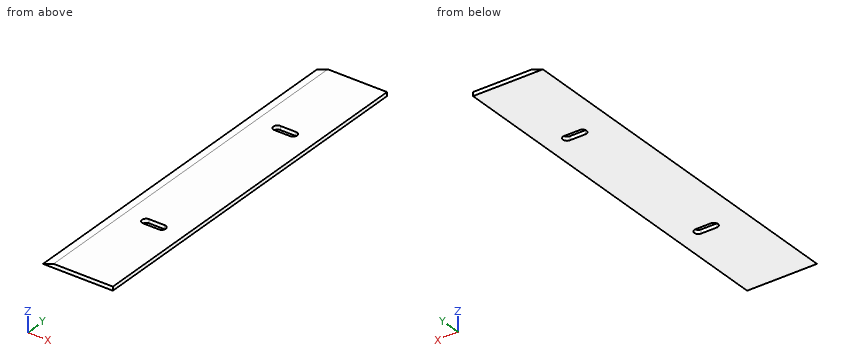
```python
from build123d import *

# Parameters (mm, degrees)
SKETCH_1_W          = 18
SKETCH_1_H          = 96
EXTRUDE_1_DEPTH     = 1
CUT_EXTRUDE_1_DEPTH = 117.756631965


with BuildPart() as part:
    # Эскиз1 → Бобышка-Вытянуть1 (new body)
    with BuildSketch(Plane.XY):
        with Locations((-57.446302439, 0)):
            Rectangle(SKETCH_1_W, SKETCH_1_H)
        with BuildLine():
            Line((-54.254431019, 21.962877229), (-58.271972276, 21.962877229))
            ThreePointArc((-58.271972276, 21.962877229), (-59.309095047, 23), (-58.271972276, 24.037122771))
            Line((-58.271972276, 24.037122771), (-54.254431019, 24.037122771))
            ThreePointArc((-54.254431019, 24.037122771), (-53.217308248, 23), (-54.254431019, 21.962877229))
        make_face(mode=Mode.SUBTRACT)
        with BuildLine():
            Line((-54.254431019, -21.962877229), (-58.271972276, -21.962877229))
            ThreePointArc((-58.271972276, -21.962877229), (-59.309095047, -23), (-58.271972276, -24.037122771))
            Line((-58.271972276, -24.037122771), (-54.254431019, -24.037122771))
            ThreePointArc((-54.254431019, -24.037122771), (-53.217308248, -23), (-54.254431019, -21.962877229))
        make_face(mode=Mode.SUBTRACT)
    extrude(amount=EXTRUDE_1_DEPTH)

    # Эскиз2 → Вырез-Вытянуть1 (cut, through all)
    with BuildSketch(Plane(origin=(0, 48, 0), x_dir=(1, 0, 0), z_dir=(0, 1, 0))):
        Polygon((-66.446302439, 0), (-63.698825019, -1), (-66.446302439, -1), align=None)
    extrude(amount=-CUT_EXTRUDE_1_DEPTH, mode=Mode.SUBTRACT)


solid = part.part
```
Could you check a few things on this model? Use its own coordinates, in mm. Give positions to 0.01 mm unless a question says otherwise; leave off trailing zeros. Order: outer loops, then holes, each group sorted by start corner. A loop starts at its lowest first (then second) coordinate and runs counter-clockwise, first axis right, second up.
Q1. Suppose I cut it at B-B, the plane y = 23. Write out the boundary of the cut face in (x, z), and give its area (3 significant figures).
Q2. Suppose I cut it at D-D, the plane y = 10. Write out the boundary of the cut face in (x, z).
Q3. Suppose I cut it at C-C, the plane z = 0.85. Write out the boundary of the cut face in (x, y), and give its area (3 significant figures).
Q4. Suppose I cut it at A-A, the plane x = -57. Write out the boundary of the cut face in (y, z).
Q5. If I drill on line 1 along Y through (x, z) = (-56.25, 0.6); line 2 along Z through (x, y) = (-65, 23.5), over which ranges is the centre line in solid material (lowest first)?
Solution:
1. outline: (-66.45, 0) - (-59.31, 0) - (-59.31, 1) - (-63.7, 1) - close; (-53.22, 0) - (-48.45, 0) - (-48.45, 1) - (-53.22, 1) - close
1. area: 10.5 mm2
2. outline: (-66.45, 0) - (-48.45, 0) - (-48.45, 1) - (-63.7, 1) - close
3. outline: (-64.11, -48) - (-48.45, -48) - (-48.45, 48) - (-64.11, 48) - close; hole (-58.27, -24.04) - (-54.25, -24.04) arc R1.04 ccw to (-54.25, -21.96) - (-58.27, -21.96) arc R1.04 ccw to start; hole (-58.27, 21.96) - (-54.25, 21.96) arc R1.04 ccw to (-54.25, 24.04) - (-58.27, 24.04) arc R1.04 ccw to start
3. area: 1,480 mm2
4. outline: (-48, 0) - (-24.04, 0) - (-24.04, 1) - (-48, 1) - close; (-21.96, 0) - (21.96, 0) - (21.96, 1) - (-21.96, 1) - close; (24.04, 0) - (48, 0) - (48, 1) - (24.04, 1) - close
5. line 1: y = -48 to -24.04, -21.96 to 21.96, 24.04 to 48
5. line 2: z = 0 to 0.53
